from build123d import *

# Parameters (mm, degrees)
BOSS_EXTRUDE1_DEPTH      = 1.5
SKETCH5_W                = 13
SKETCH5_H                = 1.2
BOSS_EXTRUDE2_DEPTH      = 0.8
CHAMFER1_SIZE            = 0.5
SKETCH6_R                = 10
CUT_EXTRUDE3_DEPTH       = 1.5
CHAMFER1_OF_MIRROR1_SIZE = 0.5
CUT_EXTRUDE1_REACH       = 3.5
FILLET1_R                = 4.6


with BuildPart() as part:
    # Sketch1 → Boss-Extrude1 (new body)
    with BuildSketch(Plane.XY):
        Polygon((0, 22.557357671), (25.107179677, 37.052994616), (64.834314575, 37.052994616), (101.434314575, 0.452994616), (89.834314575, -11.147005384), (20.107179677, -11.147005384), (0, 0.461880215), align=None)
    boss_extrude1 = extrude(amount=BOSS_EXTRUDE1_DEPTH)

    # Sketch5 → Boss-Extrude2 (add)
    with BuildSketch(Plane(origin=(0, 0, 0), x_dir=(-1, 0, 0), z_dir=(0, 0, -1))):
        with Locations((-44.970747126, 37.652994616)):
            Rectangle(SKETCH5_W, SKETCH5_H)
        with Locations((-54.970747126, -11.747005384)):
            Rectangle(SKETCH5_W, SKETCH5_H)
        Polygon((-78.538120497, 23.349188694), (-87.730508653, 14.156800538), (-88.57903679, 15.005328676), (-79.386648635, 24.197716831), align=None)
        Polygon((-18.182754963, 33.055176144), (-6.924424714, 26.555176144), (-6.324424714, 27.594406628), (-17.582754963, 34.094406628), align=None)
    boss_extrude2 = extrude(amount=-BOSS_EXTRUDE2_DEPTH)

    # Chamfer1
    chamfer1_edges = [part.edges().sort_by_distance(p)[0] for p in [
        (44.970747126, 38.252994616, 0),
        (54.970747126, -12.347005384, 0),
        (83.982842712, 19.601522754, 0),
        (11.953589838, 30.844406628, 0),
    ]]
    chamfer(chamfer1_edges, length=CHAMFER1_SIZE)

    # Sketch6 → Cut-Extrude3 (cut)
    with BuildSketch(Plane.XY.offset(1.5)):
        with Locations((101.434314575, 0.452994616)):
            Circle(SKETCH6_R)
    cut_extrude3 = extrude(amount=-CUT_EXTRUDE3_DEPTH, mode=Mode.SUBTRACT)

    # Mirror1: Boss-Extrude1, Boss-Extrude2, Cut-Extrude3 across plane
    add(boss_extrude1.mirror(Plane(origin=(0, 0.461880215, 1.5), x_dir=(0, 0, 1), z_dir=(1, 0, 0))))
    add(boss_extrude2.mirror(Plane(origin=(0, 0.461880215, 1.5), x_dir=(0, 0, 1), z_dir=(1, 0, 0))))
    add(cut_extrude3.mirror(Plane(origin=(0, 0.461880215, 1.5), x_dir=(0, 0, 1), z_dir=(1, 0, 0))), mode=Mode.SUBTRACT)

    # Chamfer1 of Mirror1
    chamfer1_of_mirror1_edges = [part.edges().sort_by_distance(p)[0] for p in [
        (-44.970747126, 38.252994616, 0),
        (-54.970747126, -12.347005384, 0),
        (-83.982842712, 19.601522754, 0),
        (-11.953589838, 30.844406628, 0),
    ]]
    chamfer(chamfer1_of_mirror1_edges, length=CHAMFER1_OF_MIRROR1_SIZE)

    # Sketch2 → Cut-Extrude1 (cut, up to next)
    with BuildSketch(Plane.XY.offset(1.5), mode=Mode.PRIVATE) as cut_extrude1_sk1:
        Polygon((11.4, 7.2), (-11.4, 7.2), (-11.4, 12.8), (-5, 12.8), (-5, 14.8), (5, 14.8), (5, 12.8), (11.4, 12.8), align=None)
    cut_extrude1_tool1 = extrude(cut_extrude1_sk1.sketch, amount=-CUT_EXTRUDE1_REACH, mode=Mode.PRIVATE) & part.part
    add(cut_extrude1_tool1.solids().sort_by_distance((0, 10.514626, 1.5))[0], mode=Mode.SUBTRACT)

    # Fillet1
    fillet1_edges = [part.edges().sort_by_distance(p)[0] for p in [
        (94.363246763, 7.524062428, 0.75),
        (-25.107179677, 37.052994616, 0.75),
        (-64.834314575, 37.052994616, 0.75),
        (-89.834314575, -11.147005384, 0.75),
        (-20.107179677, -11.147005384, 0.75),
        (64.834314575, 37.052994616, 0.75),
        (89.834314575, -11.147005384, 0.75),
        (20.107179677, -11.147005384, 0.75),
        (25.107179677, 37.052994616, 0.75),
        (-94.363246763, 7.524062428, 0.75),
        (-94.363246763, -6.618073196, 0.75),
        (94.363246763, -6.618073196, 0.75),
    ]]
    fillet(fillet1_edges, radius=FILLET1_R)


solid = part.part
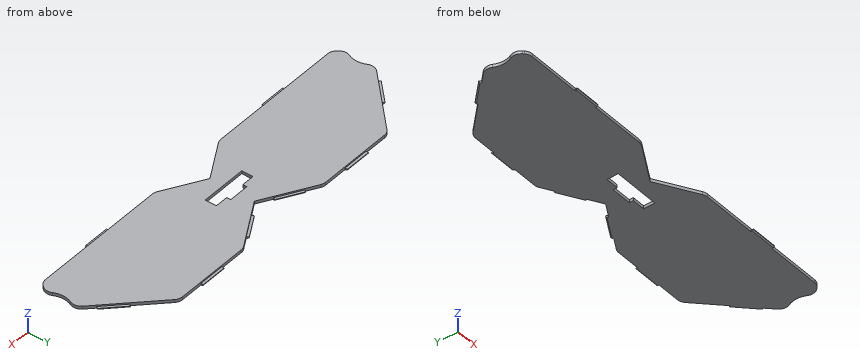
Could you check a few things on this model? Use its own coordinates, in mm. Round coordinates to 2 decimals unless told otherwise and drop trailing zeros. Write each loop counter-clockwise with the first axis right and the second up, starting at its lowest first coordinate (ties: lowest second). Pieces come first, ordered by that corner, then holes. Notation, with made-up numbers: (34.5, -23.75) - (62.5, -23.75) arc R10 cw to (62.5, -12.75) - close; hole circle Ø9 at (-1.5, 12.25). An arc over 180 degrees is marked (long way). Use a Markdown table: item, result.
Q1. I want a section at A-A (y = -1.5). List the corners of the cut face in (x, z) for me.
Output values:
| item | result |
|---|---|
| outline | (-91.63, 0) - (-3.4, 0) - (-3.4, 1.5) - (-91.63, 1.5) - close; (3.4, 0) - (91.63, 0) - (91.63, 1.5) - (3.4, 1.5) - close |
Q2. Please list where these lines run through material, in increasing order: L1, parallel to X at y = 9, z = 1.35; L2, parallel to Y at x = 44, z = 1.2; L3, parallel to X at y = 5, z = 0.1.
Output values:
| item | result |
|---|---|
| L1 | -92.53 to -11.4, 11.4 to 92.53 |
| L2 | -11.15 to 37.05 |
| L3 | -92.53 to 92.53 |
Q3. I want a section at C-C (x = -45.5). List the corners of the cut face in (y, z) for me.
Output values:
| item | result |
|---|---|
| outline | (-11.15, 0) - (37.75, 0) - (38.25, 0.5) - (38.25, 0.8) - (37.05, 0.8) - (37.05, 1.5) - (-11.15, 1.5) - close |
Q4. For pin 1 (0.6 mm diameter, centred on x = -46.5, y = 38, fed in from +Z); pin 2 (3 mm diameter, centred on x = -85, y = 17.5, fed in from +Z); pin 3 (0.8 mm diameter, centred on x = 53.5, z = 0.5, fed in from +Y), each with a flat end and sliding along its axis, tell me the tip position at first contact or that it passes through.
Output values:
| item | result |
|---|---|
| pin 1 | z = 0.8 |
| pin 2 | z = 1.5 |
| pin 3 | y = 37.05 |
